from build123d import *

# Parameters (mm, degrees)
SKETCH1_R           = 2.8
SKETCH1_R_2         = 7
SKETCH1_R_3         = 1.75
BOSS_EXTRUDE1_DEPTH = 10
SKETCH2_R           = 30
SKETCH2_R_2         = 18.7
BOSS_EXTRUDE2_DEPTH = 10
BOSS_EXTRUDE3_DEPTH = 15
FILLET1_R           = 10
FILLET2_R           = 6
SKETCH4_R           = 2.85
CUT_EXTRUDE1_DEPTH  = 30
BOSS_EXTRUDE4_DEPTH = 5
CHAMFER1_SIZE       = 2.5
CHAMFER2_SIZE       = 2.5


with BuildPart() as part:
    # Sketch1 → Boss-Extrude1 (new body)
    with BuildSketch(Plane(origin=(0, 0, 0), x_dir=(1, 0, 0), z_dir=(0, 1, 0))):
        with BuildLine():
            Line((-20, -39), (20, -39))
            Line((20, -39), (20, 5.000681491))
            Line((20, 5.000681491), (27.896886999, 24.965633249))
            ThreePointArc((27.896886999, 24.965633249), (-0.000134778, 65.999951351), (-27.897156555, 24.965633249))
            Line((-27.897156555, 24.965633249), (-20, 5))
            Line((-20, 5), (-20, -39))
        make_face()
        with Locations(Location((0, -29, 0), (0, 0, 270))):
            Circle(SKETCH1_R, mode=Mode.SUBTRACT)
        with Locations(Location((0, 42.999802972, 0), (0, 0, 270))):
            Circle(SKETCH1_R_2, mode=Mode.SUBTRACT)
        with Locations(Location((15.499926834, 35.999990173, 0), (0, 0, 270))):
            Circle(SKETCH1_R_3, mode=Mode.SUBTRACT)
        with Locations(Location((7.74993935, 22.576589188, 0), (0, 0, 270))):
            Circle(SKETCH1_R_3, mode=Mode.SUBTRACT)
        with Locations(Location((-7.75006065, 22.576574736, 0), (0, 0, 270))):
            Circle(SKETCH1_R_3, mode=Mode.SUBTRACT)
        with Locations(Location((-15.500073166, 35.999961269, 0), (0, 0, 270))):
            Circle(SKETCH1_R_3, mode=Mode.SUBTRACT)
        with Locations(Location((-7.750085682, 49.423362253, 0), (0, 0, 270))):
            Circle(SKETCH1_R_3, mode=Mode.SUBTRACT)
        with Locations(Location((7.749914318, 49.423376705, 0), (0, 0, 270))):
            Circle(SKETCH1_R_3, mode=Mode.SUBTRACT)
        with Locations(Location((0, -4, 0), (0, 0, 270))):
            Circle(SKETCH1_R, mode=Mode.SUBTRACT)
    extrude(amount=BOSS_EXTRUDE1_DEPTH)

    # Sketch2 → Boss-Extrude2 (add)
    with BuildSketch(Plane.XZ):
        with Locations(Location((-0.000109725, -35.999802972, 0), (0, 0, 21.711201864))):
            Circle(SKETCH2_R)
        with Locations(Location((-0.000109725, -35.999802972, 0), (0, 0, 270))):
            Circle(SKETCH2_R_2, mode=Mode.SUBTRACT)
    extrude(amount=BOSS_EXTRUDE2_DEPTH)

    # Sketch3 → Boss-Extrude3 (add, symmetric)
    with BuildSketch(Plane.XY.offset(9)):
        Polygon((20, 10), (105, 10), (105, -30), (95, -30), (95, -3.535533906), (91.464466094, 0), (20, 0), align=None)
    extrude(amount=BOSS_EXTRUDE3_DEPTH, both=True)

    # Fillet1
    fillet1_edges = [part.edges().sort_by_distance(p)[0] for p in [
        (20, 5, 24),
    ]]
    fillet(fillet1_edges, radius=FILLET1_R)

    # Fillet2
    fillet2_edges = [part.edges().sort_by_distance(p)[0] for p in [
        (20.395267939, 5, -6),
    ]]
    fillet(fillet2_edges, radius=FILLET2_R)

    # Sketch4 → Cut-Extrude1 (cut)
    with BuildSketch(Plane(origin=(105, 0, 0), x_dir=(0, 0, -1), z_dir=(1, 0, 0))):
        with Locations((-9, -15)):
            Circle(SKETCH4_R)
    extrude(amount=-CUT_EXTRUDE1_DEPTH, mode=Mode.SUBTRACT)

    # Sketch5 → Boss-Extrude4 (add)
    with BuildSketch(Plane(origin=(0, 0, -6), x_dir=(-1, 0, 0), z_dir=(0, 0, -1))):
        Polygon((-95, -30), (-95, 0), (-65, 0), align=None)
    boss_extrude4 = extrude(amount=-BOSS_EXTRUDE4_DEPTH)

    # Mirror1: Boss-Extrude4 across plane
    add(boss_extrude4.mirror(Plane.XY.offset(9)))

    # Chamfer1
    chamfer1_edges = [part.edges().sort_by_distance(p)[0] for p in [
        (0, 0, 1.2),
    ]]
    chamfer(chamfer1_edges, length=CHAMFER1_SIZE)

    # Chamfer2
    chamfer2_edges = [part.edges().sort_by_distance(p)[0] for p in [
        (0, 0, 26.2),
    ]]
    chamfer(chamfer2_edges, length=CHAMFER2_SIZE)


solid = part.part
CAD build for the part. Positions are in the model's coordinates, mm. A direction names the side the tool comes from. Give positions to 0.01 mm unless a question says otherwise; leave off trailing zeros. Write each loop counter-clockwise with the first axis right and the second up, starting at its lowest first coordinate (ties: lowest second). Pieces come first, ordered by that corner, then holes. Notation, with made-up numbers: M -16.5,-34 L -4.5,-34 A21 cw -4.5,-11 Z; hole C 75.5,51 d7. An arc over 180 degrees is marked long. Put each result on its own line as item: value. Start each with the question number.
(1) Band-saw the part on C-C, the plane y = -6.5. Write the cut outline in (x, z), and give its area (3 significant figures).
(2) Band-saw the part on B-B, the plane x = 68. Write the cut outline in (y, z).
(3) Mould opens along Z. For faces 5 (the face through (0, 5, 39)), 6 (the face through (105, -10, 9)), 7 (the face through (0.878, 2.379, 6.786)) say: +Z half, -Z half, draft (parallel to the pull), parting line (faces both ways), or undercut.
(4) Flat gauge pins, fed straight in: pin 1 Ø3 at (y, z) = (-2.5, -44) entering from +X; pin 2 Ø3 at (x, y) = (75, -9) entering from +Z; pin 3 Ø15 at (x, y) = (75, -18.5) entering from -Z; pin 4 Ø8.5 at (x, z) = (0, -43) entering from +Y. Where does each tip first touch, or does it go through?
(5) Probe L1, parallel to Z at x = 87.5, y = -2; L2, parallel to Y at x = -11, z = 22.5; L3, parallel to X at y = 2.5, z = 7.5. List the from-to ranges inside material, lowest first.
(6) Band-saw the part on A-A, the plane y = -22. Write the cut outline in (x, z), and give its area (3 significant figures).
(7) Which spindle directions (+Z, -Z, +X, -X, +Y, -Y) get a long thin tool onto all of the face, cutting with end or side? Do faces 1 (the face through (-20, 5, 17)), 2 (the face through (25.74, 4.93, -19.51)), 3 (the face through (95, -17, 11.4)), 4 (the face through (0, 0, -32)). Say none if no direction does.
(8) Band-saw the part on D-D, the plane y = 5.5. Give the number of separate pieces and of enclosed holes in the cut face, and give its area (3 significant figures).
Response values:
1. outline: C 0,-36 d60; M 71.5,-6 L 105,-6 L 105,24 L 71.5,24 L 71.5,19 L 95,19 L 95,-1 L 71.5,-1 Z; hole C 0,-36 d37.4
1. area: 2,260 mm2
2. outline: M -3,-6 L 10,-6 L 10,24 L -3,24 L -3,19 L 0,19 L 0,-1 L -3,-1 Z
3. face 5: +Z half
3. face 6: draft
3. face 7: undercut
4. pin 1: stops at x = 29.29
4. pin 2: stops at z = 24
4. pin 3: stops at z = -6
4. pin 4: passes through
5. L1: z = -6 to -1, 19 to 24
5. L2: y = 0 to 10
5. L3: x = -20 to 105
6. outline: M 87,-6 L 105,-6 L 105,24 L 87,24 L 87,19 L 95,19 L 95,-1 L 87,-1 Z
6. area: 380 mm2
7. face 1: +Z, -X, +Y, -Y
7. face 2: +X, +Y, -Y
7. face 3: -X, -Y
7. face 4: -Y
8. separate pieces: 1
8. enclosed holes: 9
8. area: 7,110 mm2
